Study the drawing (mm; zero at the part's minimum x, y, z) and answer. Give positions to 0.01 mm unless a question says otherwise; leave off trailing zeros. Order: outer loops, then holes, each group sorted by start corner. A loop starts at its lowest first (then second) coordinate and runs counter-clockwise, first axis right, second up. Notation, with made-up numbers: (77.25, 42) - (115.25, 42) arc R12 ccw to (115.25, 55) - close; hole circle Ø10 at (-8.5, -22). An arc over 180 degrees is marked (long way). Write each question's results on one line, items separated by ' | '. Start each with the question number.
Q1. Flat-ended cylindrical pins translate along their axes: P1, Ø10, axis at y = 22, z = 9.5, coming from the +X side; P2, Ø6, axis at x = 33, z = 31, coming from the +Y side; P3, Ø4, axis at y = 29.5, z = 27.5, coming from the +X side. Find the tip coordinate at first contact, or state that the pin passes through.
Q2. Find the intervals of material crossed by line 1 along Z through (x, y) = (36.5, 16.5); line 2 along X through (y, z) = (52.5, 19); line 3 along Z through (x, y) = (27, 42.5), in increasing order. Write a range as from..to.
Q3. Find section B-B on z = 7.5. Give the vertices of the cut face in (x, y).
Q4. Find section A-A on x = 34. Give the vertices of the cut face in (y, z), and give its area (3 significant figures).
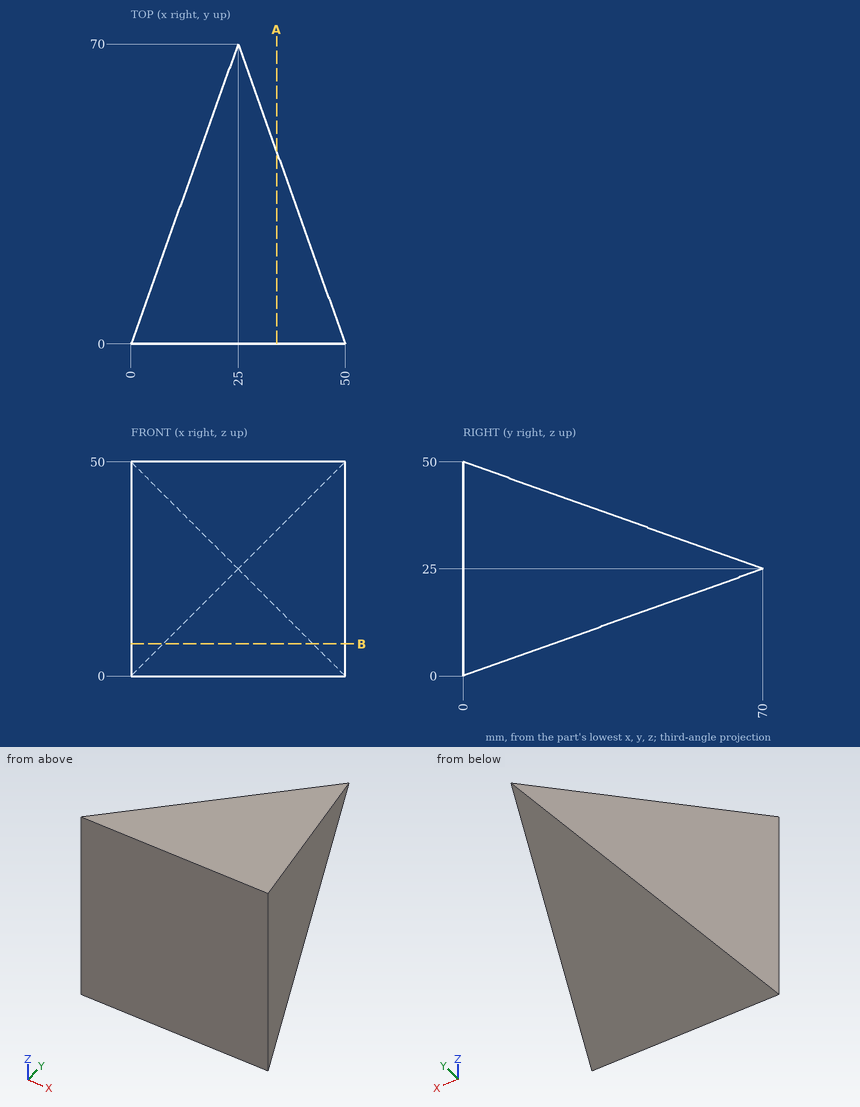
Working result:
1) P1: x = 43.93 | P2: y = 55.64 | P3: x = 40.18
2) line 1: 5.89..44.11 | line 2: 18.75..31.25 | line 3: 15.18..34.82
3) outline: (0, 0) - (50, 0) - (42.5, 21) - (7.5, 21) - close
4) outline: (0, 0) - (44.8, 16) - (44.8, 34) - (0, 50) - close | area: 1,520 mm²
